from build123d import *

# Parameters (mm, degrees)
BOSS_EXTRUDE1_START   = 505
SKETCH1_W             = 490
SKETCH1_H             = 446.8
BOSS_EXTRUDE1_DEPTH   = 3.175
FILLET1_R             = 70
EXTRUDE_THIN1_DEPTH   = 70
CUT_EXTRUDE1_DEPTH    = 10
LPATTERN1_COUNT       = 4
LPATTERN1_PITCH       = 75
SKETCH4_R             = 11.713829312
BOSS_EXTRUDE2_DEPTH   = 80
EXTRUDE_THIN3_DEPTH   = 70
EXTRUDE_THIN4_START   = -225
EXTRUDE_THIN4_DEPTH   = 3.175
EXTRUDE_THIN5_DEPTH   = 502.84
SURFACECUT4_START     = 541.993470427
SURFACECUT4_OUTLINE_W = 12
SURFACECUT4_OUTLINE_H = 409
SURFACECUT4_DEPTH     = 4.723815117


# Read off the part's stored shape, not the designer's step: Extrude-Thin3, Extrude-Thin4, SurfaceCut4
with BuildPart() as part:
    # Sketch1 → Boss-Extrude1 (new body)
    with BuildSketch(Plane.XY.offset(BOSS_EXTRUDE1_START)):
        with Locations((20, 226.6)):
            Rectangle(SKETCH1_W, SKETCH1_H)
    extrude(amount=BOSS_EXTRUDE1_DEPTH)

    # Fillet1
    fillet1_edges = [part.edges().sort_by_distance(p)[0] for p in [
        (265, 450, 506.5875),
    ]]
    fillet(fillet1_edges, radius=FILLET1_R)

    # Sketch2 → Extrude-Thin1 (add)
    with BuildSketch(Plane.XY.offset(508.175)):
        Polygon((-225, 316.632001972), (-182.911143749, 292.331989485), (-162.795993223, 327.172452198), (-160.046362566, 325.584952198), (-181.749013092, 287.994858828), (-226.5875, 313.882371315), align=None)
    extrude_thin1 = extrude(amount=EXTRUDE_THIN1_DEPTH)

    # Sketch3 → Cut-Extrude1 (cut)
    with BuildSketch(Plane(origin=(-261.017191771, 150.698345932, 0), x_dir=(0, 0, -1), z_dir=(0.86602540378444, -0.49999999999999756, 0))):
        with BuildLine():
            Line((-526.749692135, 201.941658411), (-526.749692135, 177.989368438))
            ThreePointArc((-526.749692135, 177.989368438), (-543.175, 161.564060573), (-559.600307865, 177.989368438))
            Line((-559.600307865, 177.989368438), (-559.600307865, 201.941658411))
            ThreePointArc((-559.600307865, 201.941658411), (-543.175, 218.366966275), (-526.749692135, 201.941658411))
        make_face()
    cut_extrude1 = extrude(amount=-CUT_EXTRUDE1_DEPTH, mode=Mode.SUBTRACT)

    # LPattern1: Extrude-Thin1, Cut-Extrude1 ×4
    with Locations(*[(0, -i * LPATTERN1_PITCH, 0) for i in range(1, LPATTERN1_COUNT)]):
        add(extrude_thin1)
        add(cut_extrude1, mode=Mode.SUBTRACT)

    # Sketch4 → Boss-Extrude2 (add)
    with BuildSketch(Plane.XY.offset(508.175)):
        with Locations((-35.00971575, 214.777573056)):
            Circle(SKETCH4_R)
    extrude(amount=BOSS_EXTRUDE2_DEPTH)

    # Extrude-Thin3 outline → Extrude-Thin3 (add)
    with BuildSketch(Plane.XY.offset(508.175)):
        Polygon((-225, 450), (-225, 392.649743917), (-150.706309563, 349.756261744), (-149.118809563, 352.505892401), (-221.825, 394.482831022), (-221.825, 450), align=None)
        Polygon((-225, 87.965827762), (-225, 3.2), (-221.825, 3.2), (-221.825, 86.132740658), align=None)
    extrude(amount=EXTRUDE_THIN3_DEPTH)

    # Extrude-Thin4 outline → Extrude-Thin4 (add)
    with BuildSketch(Plane.YZ.offset(EXTRUDE_THIN4_START)):
        with BuildLine():
            Line((3.2, 578.175), (449.741091008, 578.175))
            ThreePointArc((449.741091008, 578.175), (427.323091613, 623.740277235), (380, 642.159999995))
            Line((380, 642.159999995), (3.2, 642.159999995))
            Line((3.2, 642.159999995), (3.2, 578.175))
        make_face()
    extrude(amount=EXTRUDE_THIN4_DEPTH)

    # Sketch8 → Extrude-Thin5 (add)
    with BuildSketch(Plane(origin=(0, 0, 505), x_dir=(-1, 0, 0), z_dir=(0, 0, -1))):
        Polygon((-142.726543885, 3.2), (-142.726543885, 171.264978509), (-265, 171.264978509), (-265, 174.439978509), (-139.551543885, 174.439978509), (-139.551543885, 3.2), align=None)
    extrude(amount=EXTRUDE_THIN5_DEPTH)

    # SurfaceCut4 outline → SurfaceCut4 (cut)
    with BuildSketch(Plane(origin=(0, 0, 0), x_dir=(0.707106781186548, 0, -0.707106781186547), z_dir=(0.707106781186547, 0, 0.707106781186548)).offset(SURFACECUT4_START)):
        with Locations((-172, 206.5)):
            Rectangle(SURFACECUT4_OUTLINE_W, SURFACECUT4_OUTLINE_H)
    extrude(amount=SURFACECUT4_DEPTH, mode=Mode.SUBTRACT)


solid = part.part
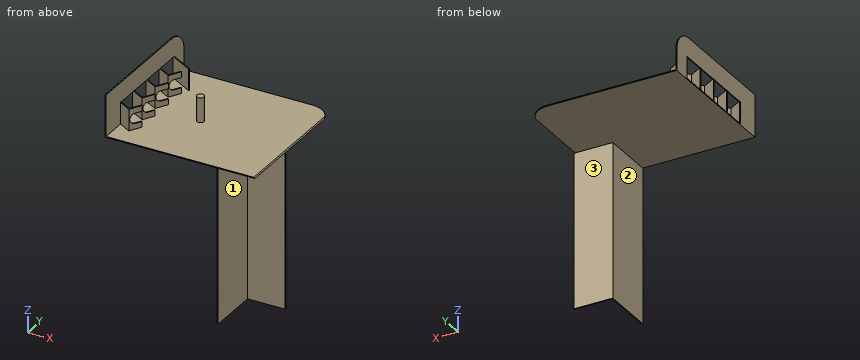
Can you work these out from the model? Positions are in its coordinate system, mm. Face numbers are marked on the shaded views. A direction names the side the tool comes from. Coordinates: 2 decimals unless noted, no trailing zeros. Write each loop counter-clockwise with the first axis right and the second up, starting at its lowest first coordinate (ties: lowest second). Pieces come first, ordered by that corner, then holes. Notation, with made-up numbers: (23.25, 56.5) - (74.25, 56.5) arc R29 ccw to (74.25, 88.5) - close; hole circle Ø10 at (-38.5, 27.25). An arc over 180 degrees is marked (long way). Return JSON: item names as keys, results as strings. Group by question number.
Item 1: If we section it at A-A (y = 274): Write out the boundary of the cut face in (x, z) (3 decimals), then the cut area to 3 significant figures.
Item 2: Which directions (+Z, -Z, +X, -X, +Y, -Y) give clear straight access to the entire face, cutting with the end or side of a thin tool? Please do the marked faces 1, 2 and 3.
Item 3: I'm going to push flat-ended pins straight in: pin 1 Ø1.3 at (x, y) = (-226, 315.5) entering from +Z (3 decimals); pin 2 Ø1 at (x, y) = (-223.5, 205) entering from -Z; pin 3 Ø1 at (x, z) = (191, 264) entering from +Y. Where does each tip first touch, or does it pass through?
Item 4: If we section it at B-B (z = 74.5): Write out the boundary of the cut face in (x, y).
Item 5: If we section it at C-C (x = 54): Write out the boundary of the cut face in (y, z) (3 decimals), then the cut area to 3 significant figures.
Item 6: If we section it at D-D (z = 596.5): Write out the boundary of the cut face in (x, y) (3 decimals), then the cut area to 3 significant figures.
Item 7: Please list where these lines run through material, in increasing order: probe 1 along Z at (x, y) = (-39.5, 369) (3 decimals); probe 2 along X at (y, z) = (130, 367); probe 3 along Y at (x, z) = (226.5, 242).
Return value:
{
 "1": {"outline": "(-225, 505) - (261.495, 505) - (258.32, 508.175) - (-225, 508.175) - close; (-225, 578.175) - (-221.825, 578.175) - (-221.825, 642.16) - (-225, 642.16) - close", "area": "1,740 mm^2"},
 "2": {"face 1": "-Z, +X, -Y", "face 2": "-Z, -X, +Y, -Y", "face 3": "-Z, +X, -X, +Y"},
 "3": {"pin 1": "stops at z = 578.175", "pin 2": "stops at z = 505", "pin 3": "stops at y = 174.44"},
 "4": {"outline": "(139.55, 3.2) - (142.73, 3.2) - (142.73, 171.26) - (265, 171.26) - (265, 174.44) - (139.55, 174.44) - close"},
 "5": {"outline": "(3.2, 505) - (450, 505) - (450, 508.175) - (3.2, 508.175) - close", "area": "1,420 mm^2"},
 "6": {"outline": "(-225, 3.2) - (-221.825, 3.2) - (-221.825, 445.632) - (-225, 445.632) - close", "area": "1,400 mm^2"},
 "7": {"probe 1": "z = 505 to 508.175", "probe 2": "x = 139.55 to 142.73", "probe 3": "y = 171.26 to 174.44"}
}
